```python
from build123d import *

# Parameters (mm, degrees)
SKETCH_1_W                  = 6
SKETCH_1_H                  = 25
SKETCH_2_R                  = 9.5
EXTRUDE_1_DEPTH             = 5
HOLE_WIZARD_1_6_1_6_1_D     = 1.6
HOLE_WIZARD_1_6_1_6_1_DEPTH = 6


with BuildPart() as part:
    # 스케치1 → 회전1 (revolve)
    with BuildSketch(Plane(origin=(0, 0, 0), x_dir=(-1, 0, 0), z_dir=(0, 0, -1))):
        with Locations((-8, 12.5)):
            Rectangle(SKETCH_1_W, SKETCH_1_H)
    revolve(axis=Axis((11, 0, 0), (-1, 0, 0)))

    # 스케치2 → 보스-돌출1 (add)
    with BuildSketch(Plane.ZY.offset(-5)):
        Circle(SKETCH_2_R)
    extrude(amount=EXTRUDE_1_DEPTH)

    # Ø1.6 (1.6) 지름 구멍1
    with Locations(Plane.ZY.offset(-5)):
        with Locations((0, 20), (-20, 0), (0, -20), (20, 0)):
            Hole(HOLE_WIZARD_1_6_1_6_1_D / 2, depth=HOLE_WIZARD_1_6_1_6_1_DEPTH)


solid = part.part
```
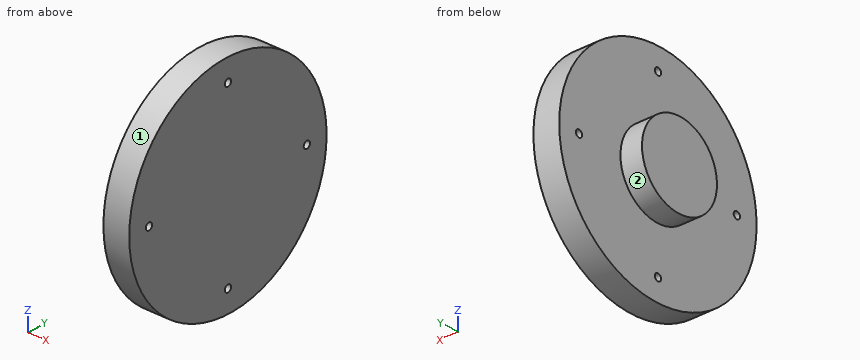
CAD build for the part. Positions are in the model's coordinates, mm. Face numbers are marked on the shaded views. A direction names the side the tool comes from. Coordinates: 2 decimals unless noted, no trailing zeros. Write each loop counter-clockwise with the first axis right and the second up, starting at its lowest first coordinate (ties: lowest second). Pieces come first, ordered by that corner, then holes. Notation, with made-up numbers: (-25, 14.25) -> (-2, 14.25) arc R13 ccw to (-2, 24.25) -> close; hole circle Ø9 at (57, 25). An arc over 180 degrees is marked (long way). Use CSV: the item, a comma, the result in double quotes. Start each with the question number.
Item 1: Band-saw the part on B-B, the plane z = 0. Write the cut outline in (x, y).
Item 2: Drop flat-ended pins along their axis: P1, Ø2, axis at x = 7.5, z = -11, coming from the +Y side; P2, Ø1.5, axis at x = 3.5, z = -12, coming from the -Y side; P3, Ø3, axis at x = 6.5, y = -3, coming from the -Z side; P4, Ø2, axis at x = 1.5, y = -1.5, coming from the +Z side. Give the stop position or say it passes through.
Item 3: Tool access for the marked faces 1 and 2: list every direction of +Z, -Z, +X, -X, +Y, -Y with a clear straight run to the whole face (end or side of a thin tool).
Item 4: Band-saw the part on A-A, the plane y = -20. Write the cut outline in (x, z), plus the area to 3 significant figures.
Item 5: Wall check: probe 1 along Y at (x, z) = (9.25, 0); probe 2 along Y at (x, z) = (9, -0.5) (1 decimal); probe 3 along X at (y, z) = (18.5, 14.5). Give the ranges that are in metal, low to high.
Response values:
1,outline,"(0, -9.5) -> (5, -9.5) -> (5, -19.2) -> (11, -19.2) -> (11, 19.2) -> (5, 19.2) -> (5, 9.5) -> (0, 9.5) -> close; (5, -25) -> (11, -25) -> (11, -20.8) -> (5, -20.8) -> close; (5, 20.8) -> (11, 20.8) -> (11, 25) -> (5, 25) -> close"
2,P1,"stops at y = 22.91"
2,P2,"passes through"
2,P3,"stops at z = -24.95"
2,P4,"stops at z = 9.49"
3,face 1,"+X, -X"
3,face 2,"-X"
4,outline,"(5, -15) -> (11, -15) -> (11, -0.8) -> (5, -0.8) -> close; (5, 0.8) -> (11, 0.8) -> (11, 15) -> (5, 15) -> close"
4,area,"170 mm2"
5,probe 1,"y = -25 to -20.8, -19.2 to 19.2, 20.8 to 25"
5,probe 2,"y = -25 to -20.6, -19.4 to 19.4, 20.6 to 25"
5,probe 3,"x = 5 to 11"
